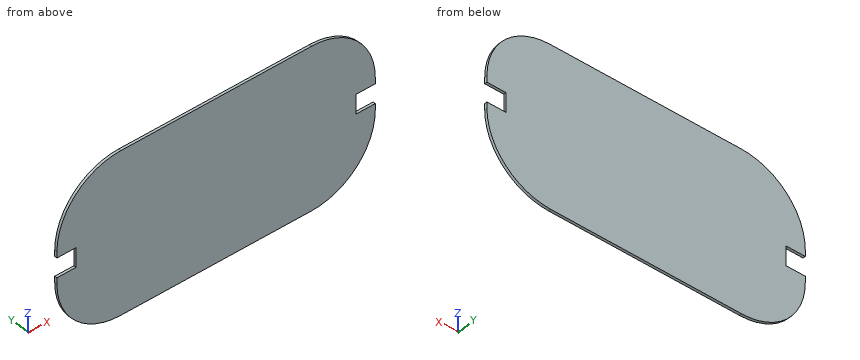
from build123d import *

# Parameters (mm, degrees)
SKETCH1_W           = 500
SKETCH1_H           = 250
BOSS_EXTRUDE1_DEPTH = 4
FILLET1_R           = 100
CUT_EXTRUDE1_DEPTH  = 10


with BuildPart() as part:
    # Sketch1 → Boss-Extrude1 (new body)
    with BuildSketch(Plane(origin=(0, 0, 0), x_dir=(1, 0, 0), z_dir=(0, 1, 0))):
        Rectangle(SKETCH1_W, SKETCH1_H)
    extrude(amount=BOSS_EXTRUDE1_DEPTH)

    # Fillet1
    fillet1_edges = [part.edges().sort_by_distance(p)[0] for p in [
        (250, 2, 125),
        (-250, 2, 125),
        (-250, 2, -125),
        (250, 2, -125),
    ]]
    fillet(fillet1_edges, radius=FILLET1_R)

    # Sketch2 → Cut-Extrude1 (cut)
    with BuildSketch(Plane(origin=(0, 0, 0), x_dir=(-1, 0, 0), z_dir=(0, -1, 0))):
        Polygon((250, 0), (250, -15), (220, -15), (220, 15), (250, 15), align=None)
        Polygon((-250, 0), (-250, -15), (-220, -15), (-220, 15), (-250, 15), align=None)
    extrude(amount=-CUT_EXTRUDE1_DEPTH, mode=Mode.SUBTRACT)


solid = part.part
CAD build for the part. Positions are in the model's coordinates, mm. Give positions to 0.01 mm unless a question says otherwise; leave off trailing zeros. Loops run counter-clockwise (first coordinate to the right, second up) from the corner with the lowest first, then second, coordinate; pieces in that order, holes last. Notation, with made-up numbers: M -30,22.5 L 12,22.5 A20 cw 12,50.5 Z; hole C 69.25,71.25 d4. An arc over 180 degrees is marked long. Write each question's results on one line, items separated by ' | '.
Q1. Band-saw the part on C-C on x = -210. Write the cut outline in (y, z), and give its area (3 significant figures).
Geometry check:
outline: M 0,-105 L 4,-105 L 4,105 L 0,105 Z | area: 840 mm²
Q2. Probe probe 1 along Z at (x, y) = (-227, 2.7); probe 2 along X at (y, z) = (0.5, 29.5); probe 3 along X at (y, z) = (0.2, 3.5). List the from-to ranges inside material, lowest first.
Geometry check:
probe 1: z = -88.8 to -15, 15 to 88.8 | probe 2: x = -249.9 to 249.9 | probe 3: x = -220 to 220
Q3. Band-saw the part on B-B on z = -82. Write the cut outline in (x, y).
Geometry check:
outline: M -232.16,0 L 232.16,0 L 232.16,4 L -232.16,4 Z
Q4. Band-saw the part on A-A on y = 0.65. Write the cut outline in (x, z).
Geometry check:
outline: M -250,-25 A100 ccw -150,-125 L 150,-125 A100 ccw 250,-25 L 250,-15 L 220,-15 L 220,15 L 250,15 L 250,25 A100 ccw 150,125 L -150,125 A100 ccw -250,25 L -250,15 L -220,15 L -220,-15 L -250,-15 Z
Q5. Flat gauge pins, fed straight in: P1, Ø2, axis at x = 239, y = 1.5, coming from the +Z side; P2, Ø1.2, axis at x = -241, y = 2.5, coming from the +Z side; P3, Ø1.2, axis at y = 2, z = -1.5, coming from the +X side. Where does each tip first touch, or does it go through?
Geometry check:
P1: stops at z = 72.5 | P2: stops at z = 67.75 | P3: stops at x = 220
